Work out the finished part from the listing and answer in its coordinate system (mm). Face numbers are marked on the shaded views. A direction names the side the tool comes from. Round coordinates to 2 decimals unless told otherwise and drop trailing zeros. Loops run counter-clockwise (first coordinate to the right, second up) from the corner with the lowest first, then second, coordinate; pieces in that order, holes last. Notation, with made-up numbers: (33, 14.25) - (89, 14.25) arc R21 ccw to (89, 32.25) - close; hole circle Ø8 at (-4.75, 44). An arc over 180 degrees is marked (long way). Answer as CSV lines item,"result". Start each with the question number.
Q1. Section D-D on z = 0.75 is taken. Write down the section's boundary in (x, y) (3 decimals).
Q2. Section C-C on y = 7.62 is taken. Write down the section's boundary in (x, z).
Q3. Each of these flat-tipped pins is pushed along its axis until it touches: pin 1 Ø6 at (x, y) = (8.5, 40.5) entering from -Z; pin 2 Ø5 at (y, z) = (28, -8.5) entering from +X. Where does it stop, or does it pass through?
Q4. Straight lines are drawn through the part: L1, parallel to X at y = 44.45, z = 1.35; L2, parallel to X at y = 57.15, z = 1.15; L3, parallel to Z at x = 13, y = 32. For each, find the intervals that lie inside material, in ascending order. Write a range as [from, to].
Q5. For the marked faces 1 and 2, determine the directions among +Z, -Z, +X, -X, +Y, -Y from which every point of the face is accessible in a straight line to the end or side of a thin tool.
Q6. Section A-A on y = 44.45 is taken. Write down the section's boundary in (x, z).
Q7. Section B-B on x = 25 is taken. Write down the section's boundary in (y, z), then the cut area to 3 significant figures.
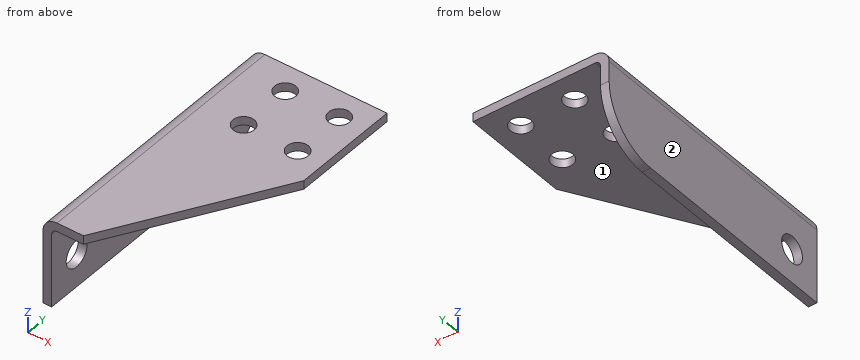
Autodesk Inventor part; units mm, degrees
ref_plane "YZ Plane" through (0, 0, 0) normal (1, 0, 0) x (0, 1, 0)
ref_plane "XZ Plane" through (0, 0, 0) normal (0, 1, 0) x (-1, 0, 0)
ref_plane "XY Plane" through (0, 0, 0) normal (0, 0, 1) x (1, 0, 0)
sketch "Sketch1" plane through (0, 0, 0) normal (0, 0, 1) x (1, 0, 0)
  line L0 (0, 0) -> (32.0167, 0)
  line L1 (32.0167, 0) -> (32.0167, 63.5)
  line L2 (32.0167, 63.5) -> (0, 63.5)
  line L3 (0, 63.5) -> (0, 0)
  dimension "d0" = 63.5
  dimension "d1" = 32.0167
extrude "Plate1" add sketch "Sketch1" along normal blind 2.032
sketch "Sketch2" plane through (2.032, 63.5, 2.032) normal (-1, 0, 0) x (0, -1, 0)
  line L0 (63.5, 0) -> (0, 0)
  line L1 (0, 0) -> (0, -20.6375)
  line L2 (0, -20.6375) -> (63.5, -20.6375)
  line L3 (63.5, -20.6375) -> (63.5, 0)
edge flange "Flange1" height 20.6375 angle 90 thickness 2.032 bend radius 1.27 thickness toward (-1, 0, 0) relief tear relief width 2.032 relief depth 1.016 edges at (0, 31.75, 0) wall of the first edge with corners at (2.032, 0, 2.032) (2.032, 63.5, 2.032) (2.032, 63.5, -18.6055) (2.032, 0, -18.6055)
bend "Bend1"
corner "Corner1"
sketch "Sketch3" plane through (0, 0, 0) normal (0, 0, -1) x (-1, 0, 0)
  line L0 (-32.0167, 0) -> (-32.0167, 63.5)
  line L1 (-32.0167, 63.5) -> (-3.302, 63.5)
  point P0 (0, 0)
  point P1 (-25.6667, 57.15)
  point P2 (-12.9667, 57.15)
  point P3 (-25.6667, 44.45)
  point P4 (-12.9667, 44.45)
  dimension "d13" = 6.35
  dimension "d14" = 6.35
  dimension "d15" = 12.7
  dimension "d16" = 12.7
hole "Hole1" at (25.6667, 57.15, 0) at (12.9667, 57.15, 0) at (25.6667, 44.45, 0) at (12.9667, 44.45, 0) direction (0, 0, 1) diameter 4.9784 end through all
sketch "Sketch4" plane through (2.032, 0, -18.6055) normal (1, 0, 0) x (0, 0, -1)
  line L0 (-20.6375, 63.5) -> (-20.6375, 0)
  line L1 (-17.3355, 0) -> (0, 0)
  point P0 (-18.6055, 0)
  point P1 (-7.9375, 7.62)
  dimension "d31" = 12.7
  dimension "d32" = 7.62
hole "Hole2" at (2.032, 7.62, -10.668) direction (-1, 0, 0) diameter 6.35 end through all
fillet "Fillet1" radius 12.7 1 edges at (1.016, 63.5, -18.6055)
sketch "Sketch5" plane through (0, 0, 0) normal (0, 0, -1) x (-1, 0, 0)
  line L0 (-32.0167, 38.1) -> (-9.525, 0)
  line L1 (-32.0167, 0) -> (-3.302, 0)
  line L2 (0, 0) -> (0, 50.8)
  line L3 (-32.0167, 63.5) -> (-3.302, 63.5)
  line L4 (-32.0167, 0) -> (-32.0167, 63.5)
  line L5 (-32.0167, 38.1) -> (-32.0167, 0)
  line L6 (-32.0167, 0) -> (-9.525, 0)
  dimension "d34" = 9.525
  dimension "d35" = 25.4
extrude "Extrusion1" cut sketch "Sketch5" against normal through all
equation "\"d22\" = Thickness"
equation "\"d29\" = Thickness"
equation "\"d2\" = Thickness"
equation "\"d3\" = BendReliefWidth"
equation "\"d4\" = BendReliefDepth"
equation "\"d5\" = MinimumRemnant"
equation "\"d6\" = TransitionRadius"
equation "\"d9\" = BendRadius"
equation "\"d10\" = CornerReliefSize"
equation "\"d11\" = GapSize"
equation "\"d12\" = JacobiRadiusSize"
equation "\"BendReliefWidth\" = Thickness"
equation "\"BendReliefDepth\" = 0.5 * Thickness"
equation "\"CornerReliefSize\" = 4 * Thickness"
equation "\"MinimumRemnant\" = 2 * Thickness"
equation "\"TransitionRadius\" = BendRadius"
equation "\"JacobiRadiusSize\" = BendRadius"
equation "\"GapSize\" = Thickness"
properties part number "Roller bracket" material "Aluminum 6061"
Findings:
1,outline,"(0.69, 0) - (9.525, 0) - (32.017, 38.1) - (32.017, 63.5) - (0.69, 63.5) - close; hole circle Ø4.978 at (12.967, 44.45); hole circle Ø4.978 at (12.967, 57.15); hole circle Ø4.978 at (25.667, 44.45); hole circle Ø4.978 at (25.667, 57.15)"
2,outline,"(0, -18.61) - (2.03, -18.61) - (2.03, -13.84) - (0, -13.84) - close; (0, -7.49) - (2.03, -7.49) - (2.03, -1.27) arc R1.27 cw to (3.3, 0) - (14.02, 0) - (14.02, 2.03) - (3.3, 2.03) arc R3.3 ccw to (0, -1.27) - close"
3,pin 1,"stops at z = 0"
3,pin 2,"stops at x = 2.03"
4,L1,"x = [1.29, 10.48], [15.46, 23.18], [28.16, 32.02]"
4,L2,"x = [1.06, 10.48], [15.46, 23.18], [28.16, 32.02]"
4,L3,"z = [0, 2.03]"
5,face 1,"-Z, +X, +Y, -Y"
5,face 2,"+Z, -Z, -X, +Y, -Y"
6,outline,"(0, -18.61) - (2.03, -18.61) - (2.03, -1.27) arc R1.27 cw to (3.3, 0) - (10.48, 0) - (10.48, 2.03) - (3.3, 2.03) arc R3.3 ccw to (0, -1.27) - close; (15.46, 0) - (23.18, 0) - (23.18, 2.03) - (15.46, 2.03) - close; (28.16, 0) - (32.02, 0) - (32.02, 2.03) - (28.16, 2.03) - close"
7,outline,"(26.21, 0) - (42.05, 0) - (42.05, 2.03) - (26.21, 2.03) - close; (46.85, 0) - (54.75, 0) - (54.75, 2.03) - (46.85, 2.03) - close; (59.55, 0) - (63.5, 0) - (63.5, 2.03) - (59.55, 2.03) - close"
7,area,"56.3 mm^2"
